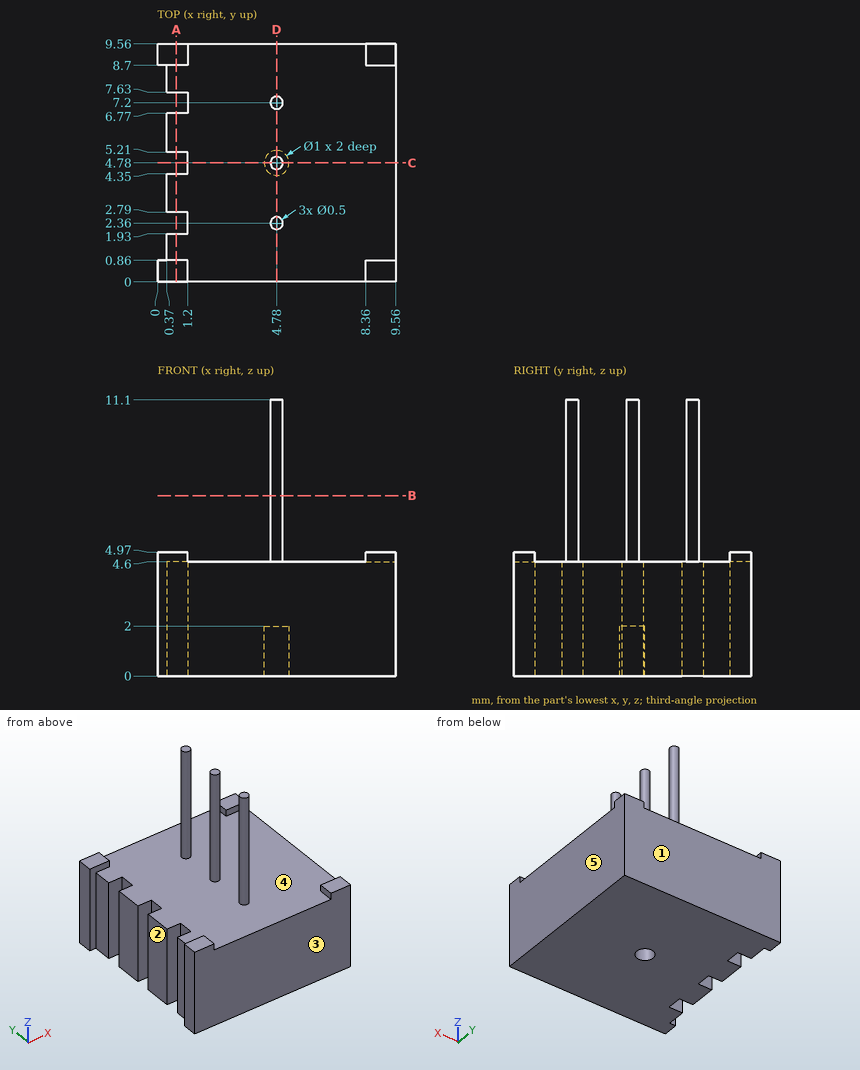
Can you work these out from the drawing? Everything is in mm from the part's minimum corner. A direction names the side the tool comes from. Round coordinates to 2 decimals unless told otherwise and drop trailing zeros. Loops run counter-clockwise (first coordinate to the right, second up) from the corner with the lowest first, then second, coordinate; pieces in that order, holes last. Notation, with made-up numbers: (25, 63) -> (83, 63) arc R23 cw to (83, 99) -> close; hole circle Ø1 at (47, 85). An arc over 180 degrees is marked (long way). Put each result on its own line as item: value.
Q1. I want a section at B-B on z = 7.25. Write out the boundary of the cut face in (x, y).
Checks:
outline: circle Ø0.5 at (4.78, 2.36); circle Ø0.5 at (4.78, 4.78); circle Ø0.5 at (4.78, 7.2)
Q2. Please list where these lines run through material, in increasing order: line 1 (Y direction, x = 4.75, z = 10); line 2 (Y direction, x = 4.78, z = 0.7); line 3 (X direction, y = 4.78, z = 1.1). Write a range as from..to.
Checks:
line 1: 2.11..2.61, 4.53..5.03, 6.95..7.45
line 2: 0..4.28, 5.28..9.56
line 3: 1.2..4.28, 5.28..9.56
Q3. I want a section at D-D on x = 4.78. Write out the boundary of the cut face in (y, z).
Checks:
outline: (0, 0) -> (4.28, 0) -> (4.28, 2) -> (5.28, 2) -> (5.28, 0) -> (9.56, 0) -> (9.56, 4.6) -> (7.45, 4.6) -> (7.45, 11.1) -> (6.95, 11.1) -> (6.95, 4.6) -> (5.03, 4.6) -> (5.03, 11.1) -> (4.53, 11.1) -> (4.53, 4.6) -> (2.61, 4.6) -> (2.61, 11.1) -> (2.11, 11.1) -> (2.11, 4.6) -> (0, 4.6) -> close
Q4. I want a section at C-C on y = 4.78. Write out the boundary of the cut face in (x, z), and give its area (3 significant figures).
Checks:
outline: (1.2, 0) -> (4.28, 0) -> (4.28, 2) -> (5.28, 2) -> (5.28, 0) -> (9.56, 0) -> (9.56, 4.6) -> (5.03, 4.6) -> (5.03, 11.1) -> (4.53, 11.1) -> (4.53, 4.6) -> (1.2, 4.6) -> close
area: 39.7 mm2
Q5. Which directions (+Z, -Z, +X, -X, +Y, -Y) give clear straight access to the entire face, cutting with the end or side of a thin tool? Please do the marked faces 1 and 2.
Checks:
face 1: +Z, -Z, +X, -X, +Y
face 2: +Z, -Z, -X
Q6. Thinking about a two-plate mould opening in X: for the marked faces 3, 4 and 5, which applies, pulls with the +X half, pulls with the -X half, needs draft (parallel to the pull), parting line crosses it, or undercut?
Checks:
face 3: needs draft
face 4: undercut
face 5: pulls with the +X half
Q7. For pin 1 Ø0.7 at (y, z) = (7.5, 2) entering from -X; pin 2 Ø5 at (y, z) = (4.5, 9) entering from -X, each with a flat end and sliding along its axis, tell me the tip position at first contact or that it passes through.
Checks:
pin 1: x = 0.37
pin 2: x = 4.53
Q8. I want a section at A-A on x = 0.75. Write out the boundary of the cut face in (y, z).
Checks:
outline: (0, 0) -> (1.93, 0) -> (1.93, 4.6) -> (0.86, 4.6) -> (0.86, 4.97) -> (0, 4.97) -> close; (2.79, 0) -> (4.35, 0) -> (4.35, 4.6) -> (2.79, 4.6) -> close; (5.21, 0) -> (6.77, 0) -> (6.77, 4.6) -> (5.21, 4.6) -> close; (7.63, 0) -> (9.56, 0) -> (9.56, 4.97) -> (8.7, 4.97) -> (8.7, 4.6) -> (7.63, 4.6) -> close
